Work out the finished part from the listing and answer in its coordinate system (mm). A direction names the side the tool comes from. Coordinates: 2 decimals unless noted, no trailing zeros. Order: outer loops, then holes, each group sorted by start corner. A loop starts at its lowest first (then second) coordinate and runs counter-clockwise, first axis right, second up. Notation, with made-up numbers: M 86.25,-17 L 99.25,-17 A15 cw 99.25,-10 Z; hole C -32.5,15.25 d9. An arc over 180 degrees is marked long. Use a Markdown table: item, result. Add a question column.
from build123d import *

# Parameters (mm, degrees)
F1_DEPTH = 25
F0_W     = 9.020209058
F0_H     = 7.5
F2_DEPTH = 10
F3_DEPTH = 3.125
F5_R     = 2


with BuildPart() as f1:
    # F0 (on Front) → F1 (new body, symmetric)
    with BuildSketch(Plane.XZ):
        Polygon((8.75, 3.75), (-16.25, 3.75), (-16.25, -3.75), (16.25, -3.75), (16.25, 3.75), align=None)
    extrude(amount=F1_DEPTH, both=True)

    # F0 (on Front) → F2 (join, symmetric)
    with BuildSketch(Plane.XZ):
        with BuildLine():
            Line((8.75, 11.9511034528), (8.75, 3.75))
            Line((8.75, 3.75), (16.25, 3.75))
            Line((16.25, 3.75), (16.25, 11.9511034528))
            ThreePointArc((16.25, 11.9511034528), (16.8839020833, 14.6937197566), (18.6570221407, 16.88))
            Line((18.6570221407, 16.88), (23.75, 16.88))
            Line((23.75, 16.88), (23.75, 24.38))
            Line((23.75, 24.38), (16.6190961053, 24.38))
            ThreePointArc((16.6190961053, 24.38), (10.8826653541, 19.3063761006), (8.75, 11.9511034528))
        make_face()
        with Locations((28.260104529, 20.63)):
            Rectangle(F0_W, F0_H)
    extrude(amount=F2_DEPTH, both=True)

    # F0 (on Front) → F3 (join, symmetric)
    with BuildSketch(Plane.XZ):
        with BuildLine():
            add(Edge.make_bspline(
                [(-16.25, 3.75), (-8.5098091513, 18.9848486334), (3.8099950824, 23.7404676708), (16.6190961053, 24.38)],
                knots=[0, 0, 0, 0, 38.8068857135, 38.8068857135, 38.8068857135, 38.8068857135], degree=3))
            Line((-16.25, 3.75), (8.75, 3.75))
            Line((8.75, 3.75), (8.75, 11.9511034528))
            ThreePointArc((8.75, 11.9511034528), (10.8826653541, 19.3063761006), (16.6190961053, 24.38))
        make_face()
    extrude(amount=F3_DEPTH, both=True)

    # F0 (on Front) → F4 (revolve)
    with BuildSketch(Plane.XZ):
        Polygon((43.75, 26.25), (33.75, 26.25), (33.75, 24.38), (33.75, 20.625), (33.75, 16.88), (33.75, 15), (43.75, 15), align=None)
    revolve(axis=Axis((33.75, 0, 23.4375), (0, 0, 1)))

    # F5
    f5_edges = [f1.edges().sort_by_distance(p)[0] for p in [
        (-16.25, 25, 0),
        (-16.25, -25, 0),
        (16.25, -25, 0),
        (16.25, 25, 0),
    ]]
    fillet(f5_edges, radius=F5_R)


solid = f1.part
(1) A cutting plane is placed at A-A on z = 2.5. Write down the section's boundary in (x, y), plus the area to 3 significant figures.
(2) A cutting plane is placed at B-B on y = 8. Write down the section's boundary in (x, z), plus the area to 3 significant figures.
(3) Given P1, Ø6, axis at x = 6, z = 16, coming from the +Y side (3 decimals); P2, Ø15.5, axis at x = 26.5, y = 4.5, coming from the -Z side; P3, Ø1.5, axis at x = 19, z = 18.5, coming from the +Y side, each flat-ended and moving along its own axis, determine where each tip first touches the part or whether it passes through.
(4) Straight lines are drawn through the part: line 1 (X direction, y = -21.5, z = -2); line 2 (Z direction, x = 10.5, y = 23); line 3 (Z direction, x = 36.5, y = 6.5). For each, find the intervals that lie inside material, in ascending order.
(5) Which of the six approach directions +Z, -Z, +X, -X, +Y, -Y give full straight-line access (tool end or side, diameter ignored) to faces 1 (the flat face through (18, -10, 17)), 2 (the flat face through (0, 3.125, 12)), 3 (the flat face through (0, -3.125, 12))?
(6) A cutting plane is placed at C-C on x = 29. Write down the section's boundary in (y, z).
(7) The mould has two halves that part along X. Classify faces 4 (the cylindrical face through (15.68, -24.4, 0.05)), 5 (the flat face through (22, 0, 16.88)), 6 (the cylindrical face through (-15.68, 24.4, -0.05)), 7 (the flat face through (21, 0, 24.38)): pulls with the +X half, pulls with the -X half, needs draft (parallel to the pull), parting line crosses it, or undercut.
(8) A cutting plane is placed at D-D on y = 14. Write down the section's boundary in (x, z), plus the area to 3 significant figures.
From the geometry:
| question | item | result |
|---|---|---|
| 1 | outline | M -16.25,-23 A2 ccw -14.25,-25 L 14.25,-25 A2 ccw 16.25,-23 L 16.25,23 A2 ccw 14.25,25 L -14.25,25 A2 ccw -16.25,23 Z |
| 1 | area | 1,620 mm2 |
| 2 | outline | M -16.25,-3.75 L 16.25,-3.75 L 16.25,11.95 A6.25 cw 18.66,16.88 L 27.75,16.88 L 27.75,15 L 39.75,15 L 39.75,26.25 L 27.75,26.25 L 27.75,24.38 L 16.62,24.38 A13.75 ccw 8.75,11.95 L 8.75,3.75 L -16.25,3.75 Z |
| 2 | area | 596 mm2 |
| 3 | P1 | stops at y = 3.125 |
| 3 | P2 | stops at z = 15 |
| 3 | P3 | stops at y = 10 |
| 4 | line 1 | x = -16.25 to 16.25 |
| 4 | line 2 | z = -3.75 to 3.75 |
| 4 | line 3 | z = 15 to 26.25 |
| 5 | face 1 | +Z, +X, -X, -Y |
| 5 | face 2 | +Z, -X, +Y |
| 5 | face 3 | +Z, -X, -Y |
| 6 | outline | M -10,16.88 L -8.8,16.88 L -8.8,15 L 8.8,15 L 8.8,16.88 L 10,16.88 L 10,24.38 L 8.8,24.38 L 8.8,26.25 L -8.8,26.25 L -8.8,24.38 L -10,24.38 Z |
| 7 | face 4 | pulls with the +X half |
| 7 | face 5 | undercut |
| 7 | face 6 | pulls with the -X half |
| 7 | face 7 | needs draft |
| 8 | outline | M -16.25,-3.75 L 16.25,-3.75 L 16.25,3.75 L -16.25,3.75 Z |
| 8 | area | 244 mm2 |
